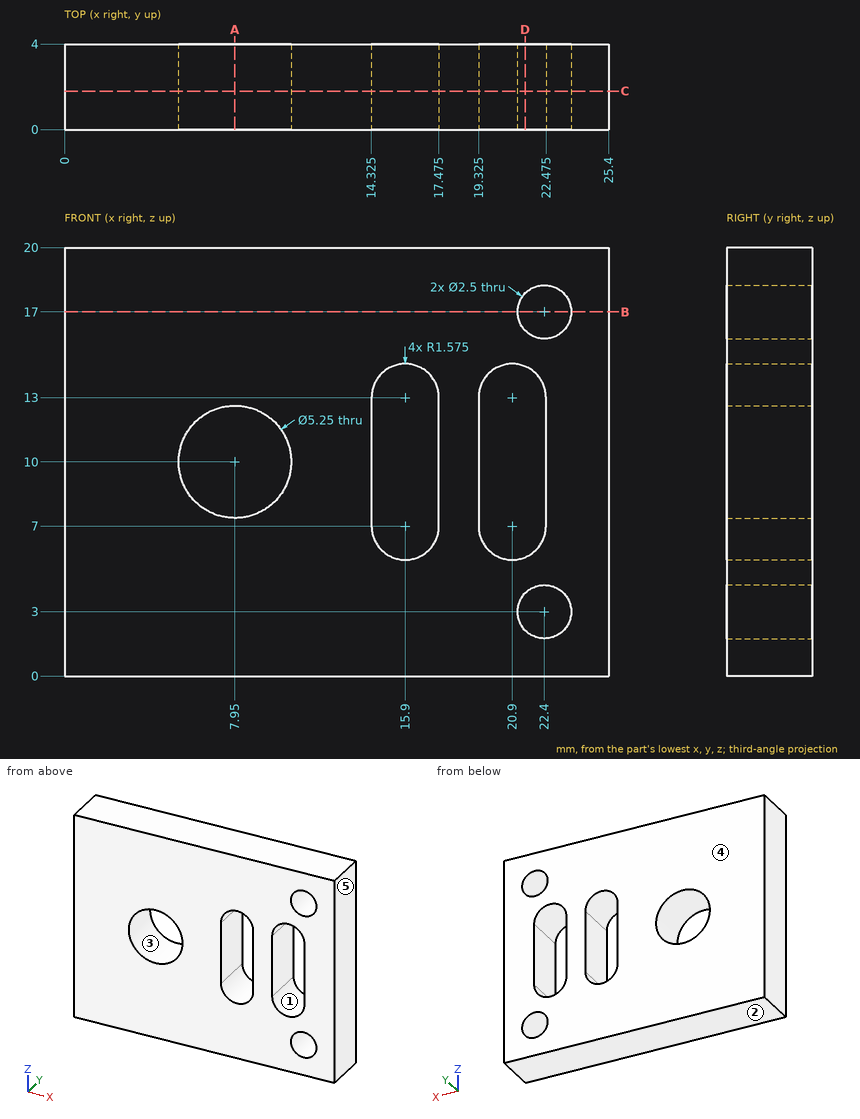
Can you work these out from the drawing? Everything is in mm from the part's minimum corner. A direction names the side the tool comes from. Round coordinates to 2 decimals unless told otherwise and drop trailing zeros. Loops run counter-clockwise (first coordinate to the right, second up) from the corner with the lowest first, then second, coordinate; pieces in that order, holes last. Notation, with made-up numbers: (88.5, 25.25) - (106.5, 25.25) arc R17 cw to (106.5, 42.25) - close; hole circle Ø6 at (68, 37). An arc over 180 degrees is marked (long way). One line per question, with ' | ' between items. Start each with the question number.
Q1. I want a section at B-B (z = 17). Write out the boundary of the cut face in (x, y).
Q2. I want a section at A-A (x = 7.95). Write out the boundary of the cut face in (y, z) (3 decimals).
Q3. For the marked faces 1 and 2, which set-ups out of +Z, -Z, +X, -X, +Y, -Y let a thin tool reach every point of the face, with its end or its side?
Q4. We'd pull the mould along X, two halves only. Please class the marked faces 3, 4 and 5: +X half, -X half, draft (parallel to the pull), parting line (faces both ways), or undercut.
Q5. I want a section at C-C (y = 1.8). Write out the boundary of the cut face in (x, z) (3 decimals).
Q6. Please list where these lines run through material, in increasing order: line 1 (X direction, y = 0.95, z = 17); line 2 (X direction, y = 2.9, z = 10) (3 decimals); line 3 (X direction, y = 3.1, z = 7.75) (3 decimals). Write a range as [from, to].
Q7. I want a section at D-D (x = 21.5). Write out the boundary of the cut face in (y, z).
Response values:
1) outline: (0, 0) - (21.15, 0) - (21.15, 4) - (0, 4) - close; (23.65, 0) - (25.4, 0) - (25.4, 4) - (23.65, 4) - close
2) outline: (0, 0) - (4, 0) - (4, 7.375) - (0, 7.375) - close; (0, 12.625) - (4, 12.625) - (4, 20) - (0, 20) - close
3) face 1: +Y, -Y | face 2: -Z, +X, -X, +Y, -Y
4) face 3: undercut | face 4: draft | face 5: +X half
5) outline: (0, 0) - (25.4, 0) - (25.4, 20) - (0, 20) - close; hole circle Ø5.25 at (7.95, 10); hole (14.325, 7) arc R1.575 ccw to (17.475, 7) - (17.475, 13) arc R1.575 ccw to (14.325, 13) - close; hole (19.325, 7) arc R1.575 ccw to (22.475, 7) - (22.475, 13) arc R1.575 ccw to (19.325, 13) - close; hole circle Ø2.5 at (22.4, 3); hole circle Ø2.5 at (22.4, 17)
6) line 1: x = [0, 21.15], [23.65, 25.4] | line 2: x = [0, 5.325], [10.575, 14.325], [17.475, 19.325], [22.475, 25.4] | line 3: x = [0, 6.598], [9.302, 14.325], [17.475, 19.325], [22.475, 25.4]
7) outline: (0, 0) - (4, 0) - (4, 2.13) - (0, 2.13) - close; (0, 3.87) - (4, 3.87) - (4, 5.54) - (0, 5.54) - close; (0, 14.46) - (4, 14.46) - (4, 16.13) - (0, 16.13) - close; (0, 17.87) - (4, 17.87) - (4, 20) - (0, 20) - close
